from build123d import *

# Parameters (mm, degrees)
F0_W     = 248
F0_H     = 176.5
F1_DEPTH = 41
F3_T     = -2.5
F4_R     = 1


with BuildPart() as f1:
    # F0 (on Top) → F1 (new body)
    with BuildSketch(Plane.XY):
        with Locations((124, 88.25)):
            Rectangle(F0_W, F0_H)
    extrude(amount=F1_DEPTH)

    # F3
    f3_openings = [f1.faces().sort_by_distance(p)[0] for p in [
        (0, 88.25, 20.5),
    ]]
    offset(amount=F3_T, openings=f3_openings)

    # F4
    f4_edges = [f1.edges().sort_by_distance(p)[0] for p in [
        (124, 176.5, 41),
        (124, 176.5, 0),
        (0, 176.5, 20.5),
        (0, 88.25, 0),
        (0, 88.25, 41),
        (124, 0, 41),
        (0, 0, 20.5),
        (124, 0, 0),
        (248, 0, 20.5),
        (248, 88.25, 41),
        (248, 88.25, 0),
        (248, 176.5, 20.5),
    ]]
    fillet(f4_edges, radius=F4_R)


solid = f1.part
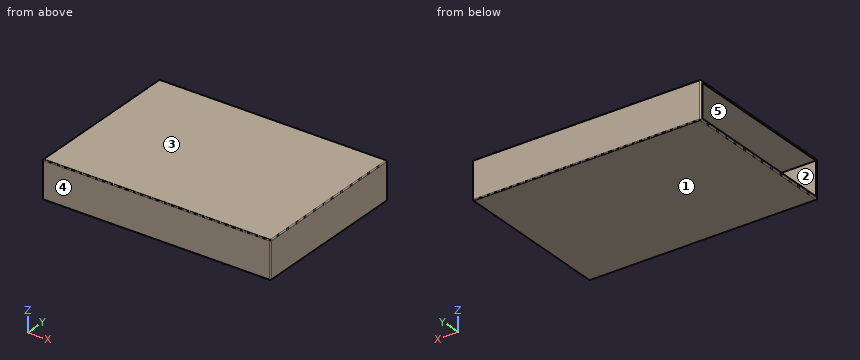
Input: part model. Units: mm. Frame: model coordinates. Face numbers are marked on the shaded views. A direction names the side the tool comes from. Round coordinates to 2 decimals unless told otherwise and drop trailing zeros. Write each loop counter-clockwise with the first axis right and the second up, starting at its lowest first coordinate (ties: lowest second). Pieces come first, ordered by that corner, then holes.
1) Cut plane A-A (x = 115.5). Return the cut outline in (y, z), then the cut area to 3 significant figures.
2) Ray query, L1, parallel to Y at x = 123, z = 3.5; L2, parallel to Z at x = 73.5, y = 78; L3, parallel to X at y = 107.5, z = 29. Return the intervals inside material, ascending.
3) Cut plane C-C (z = 12.5). Return the cut outline in (x, y), then the cut area to 3 significant figures.
4) Draft query along Y for the marked faces 3, 4 and 5. Return one class per face: pulls with the +Y half, pulls with the -Y half, needs draft (parallel to the pull), parting line crosses it, or undercut.
5) Reachability of the marked faces 1 and 2 from +Z, -Z, +X, -X, +Y, -Y: full face, straight path, thin tool, end or side. Return the list, or none.
6) Contact query for a flat-ended pin moving along its axis: P1, Ø18, axis at y = 56.5, z = 25, coming from the -X side. Output: stop coordinate, or through.
7) Cut plane B-B (y = 55). Return the cut outline in (x, z), then the cut area to 3 significant figures.
Geometry says:
1. outline: (0, 1) arc R1 ccw to (1, 0) - (175.5, 0) arc R1 ccw to (176.5, 1) - (176.5, 40) arc R1 ccw to (175.5, 41) - (1, 41) arc R1 ccw to (0, 40) - close; hole (2.5, 2.5) - (174, 2.5) - (174, 38.5) - (2.5, 38.5) - close
1. area: 1,060 mm2
2. L1: y = 0 to 2.5, 174 to 176.5
2. L2: z = 0 to 2.5, 38.5 to 41
2. L3: x = 245.5 to 248
3. outline: (0, 1) arc R1 ccw to (1, 0) - (247, 0) arc R1 ccw to (248, 1) - (248, 175.5) arc R1 ccw to (247, 176.5) - (1, 176.5) arc R1 ccw to (0, 175.5) - (0, 174) - (245.5, 174) - (245.5, 2.5) - (0, 2.5) - close
3. area: 1,670 mm2
4. face 3: needs draft
4. face 4: pulls with the -Y half
4. face 5: undercut
5. face 1: -Z, +X, -X, +Y, -Y
5. face 2: -X
6. P1: stops at x = 245.5
7. outline: (0, 1) arc R1 ccw to (1, 0) - (247, 0) arc R1 ccw to (248, 1) - (248, 40) arc R1 ccw to (247, 41) - (1, 41) arc R1 ccw to (0, 40) - (0, 38.5) - (245.5, 38.5) - (245.5, 2.5) - (0, 2.5) - close
7. area: 1,330 mm2
